Check sheet for the drawn part. Datum: minimum x, y, z corner. Units: mm. Give positions to 0.01 mm unless a question says otherwise; leave off trailing zeros. Loops run counter-clockwise (first coordinate to the right, second up) from the corner with the lowest first, then second, coordinate; pieces in that order, holes last. Notation, with made-up numbers: (83, 64.25) -> (122, 64.25) arc R21 cw to (122, 71.25) -> close; hole circle Ø5 at (70.5, 24.5). An arc over 180 degrees is marked (long way). One line per question, with ' | ' between items.
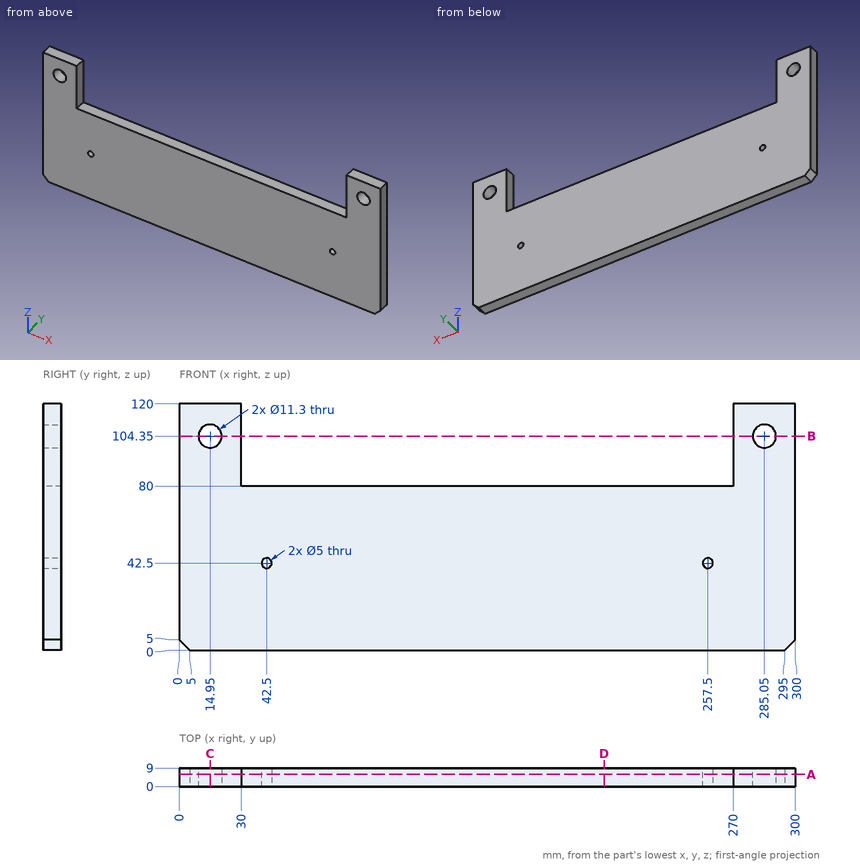
Item 1: Scan lines: probe 1 along Z at (x, y) = (285.05, 2.5); probe 2 along X at (y, z) = (8, 105); probe 3 along Z at (x, y) = (42.5, 4.75). Record each from-to range of solid material in increasing order.
Result:
probe 1: 0 to 98.7, 110 to 120 | probe 2: 0 to 9.34, 20.56 to 30, 270 to 279.44, 290.66 to 300 | probe 3: 0 to 40, 45 to 80
Item 2: Sectioned sample at B-B (z = 104.35). Record the cut outline in (x, y), plus the area to 3 significant figures.
Result:
outline: (0, 0) -> (9.3, 0) -> (9.3, 9) -> (0, 9) -> close; (20.6, 0) -> (30, 0) -> (30, 9) -> (20.6, 9) -> close; (270, 0) -> (279.4, 0) -> (279.4, 9) -> (270, 9) -> close; (290.7, 0) -> (300, 0) -> (300, 9) -> (290.7, 9) -> close | area: 337 mm2
Item 3: Sectioned sample at D-D (x = 207). Record the cut outline in (y, z), plus the area to 3 significant figures.
Result:
outline: (0, 0) -> (9, 0) -> (9, 80) -> (0, 80) -> close | area: 720 mm2
Item 4: Sectioned sample at A-A (y = 6). Record the cut outline in (x, z).
Result:
outline: (0, 5) -> (5, 0) -> (295, 0) -> (300, 5) -> (300, 120) -> (270, 120) -> (270, 80) -> (30, 80) -> (30, 120) -> (0, 120) -> close; hole circle Ø11.3 at (14.95, 104.35); hole circle Ø5 at (42.5, 42.5); hole circle Ø5 at (257.5, 42.5); hole circle Ø11.3 at (285.05, 104.35)
Item 5: Depth check by flat-ended pin: pin 1 Ø2.5 at (x, y) = (100, 6) entering from +Z. Enter the tip coordinate at first touch or a pass-through.
Result:
pin 1: z = 80
Item 6: Sectioned sample at C-C (x = 14.95). Record the cut outline in (y, z), plus the area to 3 significant figures.
Result:
outline: (0, 0) -> (9, 0) -> (9, 98.7) -> (0, 98.7) -> close; (0, 110) -> (9, 110) -> (9, 120) -> (0, 120) -> close | area: 978 mm2
